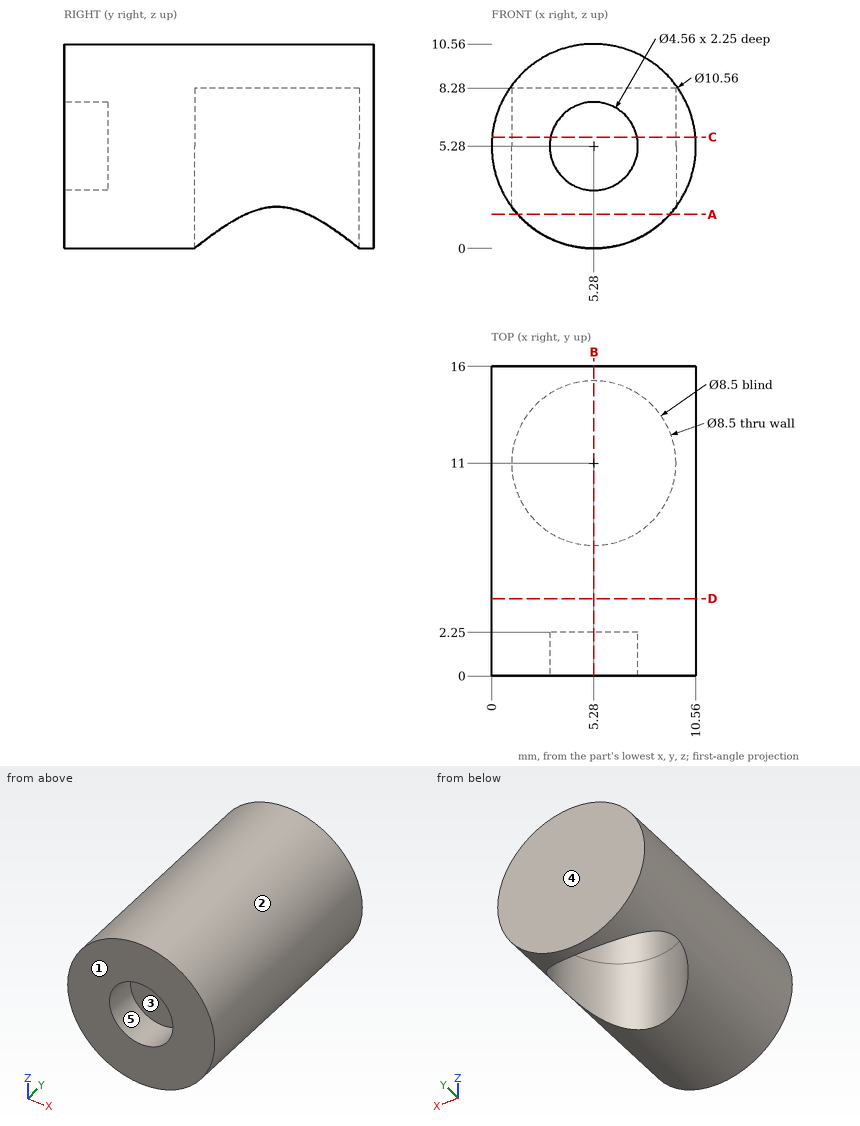
Job drawing, mm, ordinate dimensions from the low corner. One solid piece. A direction names the side the tool comes from. Give positions to 0.01 mm unless a question says otherwise; leave off trailing zeros. Loops run counter-clockwise (first coordinate to the right, second up) from the corner with the lowest first, then second, coordinate; pieces in that order, holes last. Notation, with made-up numbers: (10, 42) -> (59, 42) arc R15 cw to (59, 71) -> close; hole circle Ø4 at (75.25, -5). An arc over 180 degrees is marked (long way). Write each question's results on one line, items separated by ' | '. Start each with the question number.
Q1. Band-saw the part on C-C on z = 5.75. List the corners of the cut face in (x, y).
Q2. Band-saw the part on B-B on x = 5.28. List the corners of the cut face in (y, z), plus the area to 3 significant figures.
Q3. Band-saw the part on A-A on z = 1.75. List the corners of the cut face in (x, y), plus the area to 3 significant figures.
Q4. Wall check: L1, parallel to Z at x = 5.28, y = 1.5; L2, parallel to Y at x = 5.28, z = 4.25; L3, parallel to Y at x = 5.28, z = 1.5. Give the ranges that are in metal, low to high.
Q5. Pin check, flat tips, straight feed: P1, Ø5, axis at x = 5.28, y = 11, coming from the -Z side; P2, Ø6, axis at y = 13.5, z = 2, coming from the -X side; P3, Ø1.5, axis at x = 7.5, y = 1.5, coming from the +Z side. Stop position of each tip, or through.
Q6. Band-saw the part on D-D on y = 4. List the corners of the cut face in (x, z).
Q7. Which spindle directions (+Z, -Z, +X, -X, +Y, -Y) get a long thin tool onto all of the face, cutting with end or side? Do the marked faces 4 and 5. Say none if no direction does.
Q8. Pull direction X, two halves, no side cores. Call the marked faces 1, 2 and 3: +X half, -X half, draft (parallel to the pull), parting line (faces both ways), or undercut.
Results are:
1) outline: (0.02, 0) -> (3.05, 0) -> (3.05, 2.25) -> (7.51, 2.25) -> (7.51, 0) -> (10.54, 0) -> (10.54, 16) -> (0.02, 16) -> close; hole circle Ø8.5 at (5.28, 11)
2) outline: (0, 0) -> (6.75, 0) -> (6.75, 8.28) -> (15.25, 8.28) -> (15.25, 0) -> (16, 0) -> (16, 10.56) -> (0, 10.56) -> (0, 7.56) -> (2.25, 7.56) -> (2.25, 3) -> (0, 3) -> close | area: 88.3 mm²
3) outline: (1.35, 0) -> (9.21, 0) -> (9.21, 9.37) arc R4.25 cw to (1.35, 9.37) -> close; (1.35, 12.63) arc R4.25 cw to (9.21, 12.63) -> (9.21, 16) -> (1.35, 16) -> close | area: 70.3 mm²
4) L1: z = 0 to 3, 7.56 to 10.56 | L2: y = 2.25 to 6.75, 15.25 to 16 | L3: y = 0 to 6.75, 15.25 to 16
5) P1: stops at z = 8.28 | P2: stops at x = 0.01 | P3: stops at z = 10.35
6) outline: circle Ø10.56 at (5.28, 5.28)
7) face 4: +Z, -Z, +X, -X, +Y | face 5: -Y
8) face 1: draft | face 2: parting line | face 3: undercut
